Build history of the part. All positions in model axes, mm. A direction names the side the tool comes from. Give positions to 0.01 mm unless a question says otherwise; leave off trailing zeros. Write each loop counter-clockwise with the first axis right and the second up, starting at its lowest first coordinate (ties: lowest second). Pieces come first, ordered by that corner, then holes. Notation, with made-up numbers: M 25.5,87.25 L 35.5,87.25 A16 ccw 35.5,113.25 Z; hole C 32.25,31.5 d5. An arc over 180 degrees is marked long. Return JSON: item names as keys, results as strings. Group by question number.
Q1. Band-saw the part on B-B, the plane x = 36.5. Give the cut face in (y, z), then the cut area to 3 significant figures.
Q2. Tool access for faces 1 (the flat face through (103, 47, -1)), 2 (the flat face through (47, 8, -63)), 3 (the flat face through (105.81, 27.69, -66.84)): list every direction of +Z, -Z, +X, -X, +Y, -Y with a clear straight run to the whole face (end or side of a thin tool).
Q3. Band-saw the part on C-C, the plane z = -31.5. Give the cut face in (x, y), then the cut area to 3 significant figures.
Q4. Band-saw the part on A-A, the plane z = -13. Give the cut face in (x, y), then the cut area to 3 significant figures.
Q5. Band-saw the part on D-D, the plane z = 3.5. Give the cut face in (x, y), then the cut area to 3 significant figures.
Q6. Wall check: probe 1 along Z at (x, y) = (2, 9); probe 2 along X at (y, z) = (8.5, -52.5); probe 3 along Z at (x, y) = (85, 33). Give the ranges that are in metal, low to high.
Q7. Flat gauge pins, fed straight in: pin 1 Ø4 at (x, z) = (95, -59.01) entering from +Y; pin 2 Ø2 at (y, z) = (1, -43) entering from +X; pin 3 Ø6 at (x, z) = (44, -48) entering from -Y. Where does each tip first touch, or does it go through?
Q8. Pull direction X, two halves, no side cores. Call faces 4 (the flat face through (-11.06, 27.692, 1.698)), 5 (the flat face through (0, 3, -6)), 6 (the flat face through (37, 50, 2)), 7 (the flat face through (104.581, 3.042, -0.864)): +X half, -X half, draft (parallel to the pull), parting line (faces both ways), or undercut.
Autodesk Inventor part; units mm, degrees
ref_plane "YZ Plane" through (0, 0, 0) normal (1, 0, 0) x (0, 1, 0)
ref_plane "XZ Plane" through (0, 0, 0) normal (0, 1, 0) x (-1, 0, 0)
ref_plane "XY Plane" through (0, 0, 0) normal (0, 0, 1) x (1, 0, 0)
sketch "Sketch1" plane through (0, 0, 0) normal (0, 1, 0) x (-1, 0, 0)
  line L0 (0, 0) -> (-95, 0)
  line L1 (-95, 0) -> (-95, -65)
  line L2 (-95, -65) -> (0, -65)
  line L3 (0, -65) -> (0, 0)
  line L4 (0, -65) -> (12.9904, -57.5)
  line L5 (12.9904, -57.5) -> (12.9904, -7.5)
  line L6 (12.9904, -7.5) -> (0, 0)
  line L7 (-95, -65) -> (-107.9904, -57.5)
  line L8 (-107.9904, -57.5) -> (-107.9904, -7.5)
  line L9 (-107.9904, -7.5) -> (-95, 0)
  dimension "d0" = 95
  dimension "d1" = 65
  dimension "d2" = 15
  dimension "d3" = 15
  dimension "d4" = 120
  dimension "d5" = 15
  dimension "d6" = 15
  dimension "d7" = 120
extrude "Extrusion1" add sketch "Sketch1" along normal blind 5
sketch "Sketch2" plane through (0, 5, 0) normal (0, 1, 0) x (1, 0, 0)
  line L0 (1.0001, 63.5) -> (94.0001, 63.5)
  line L1 (94.0001, 63.5) -> (94.0001, 1.5)
  line L2 (94.0001, 1.5) -> (1.0001, 1.5)
  line L3 (1.0001, 1.5) -> (1.0001, 63.5)
  line L4 (0, 0) -> (95, 0)
  line L5 (-12.9904, 57.5) -> (-12.9904, 7.5)
  dimension "d10" = 93
  dimension "d11" = 62
  dimension "d12" = 1.5
  dimension "d13" = 13.9905
extrude "Extrusion2" add sketch "Sketch2" along normal blind 14
sketch "Sketch4" plane through (0, 5, 0) normal (0, 1, 0) x (1, 0, 0)
  line L0 (-12.9904, 57.5) -> (-12.9904, 7.5)
  line L1 (-12.9904, 57.5) -> (-12.9904, 7.5)
  line L2 (-12.9904, 7.5) -> (0, 0)
  line L3 (0, 0) -> (95, 0)
  line L4 (95, 0) -> (107.9904, 7.5)
  line L5 (95, 0) -> (107.9904, 7.5)
  line L6 (107.9904, 7.5) -> (107.9904, 57.5)
  line L7 (107.9904, 57.5) -> (95, 65)
  line L8 (107.9904, 57.5) -> (95, 65)
  line L9 (95, 65) -> (0, 65)
  line L10 (95, 65) -> (0, 65)
  line L11 (0, 65) -> (-12.9904, 57.5)
  line L12 (-19.9904, 61.5415) -> (-19.9904, 3.4585)
  line L13 (114.9904, 61.5415) -> (114.9904, 3.4585)
  line L14 (-1.8756, 72) -> (96.8756, 72)
  line L15 (-19.9904, 61.5415) -> (-1.8756, 72)
  line L16 (96.8756, 72) -> (114.9904, 61.5415)
  line L17 (114.9904, 3.4585) -> (96.8756, -7)
  line L18 (-19.9904, 3.4585) -> (-1.8756, -7)
  line L19 (-1.8756, -7) -> (96.8756, -7)
  line L20 (95, 0) -> (107.9904, 7.5)
  line L21 (107.9904, 7.5) -> (107.9904, 57.5)
  line L22 (0, 0) -> (95, 0)
  dimension "d22" = 7
  dimension "d23" = 7
  dimension "d24" = 7
  dimension "d25" = 7
  dimension "d26" = 7
  dimension "d27" = 7
  dimension "d28" = 7
  dimension "d29" = 7
extrude "Extrusion4" add sketch "Sketch4" along normal blind 45 and the other way blind 5
sketch "Sketch5" plane through (0, 0, 0) normal (0, -1, 0) x (1, 0, 0)
  line L0 (2.4999, -63) -> (92.4999, -63)
  line L1 (92.4999, -63) -> (92.4999, -2)
  line L2 (92.4999, -2) -> (2.4999, -2)
  line L3 (2.4999, -2) -> (2.4999, -63)
  line L4 (0, 0) -> (95, 0)
  line L5 (-12.9904, -57.5) -> (-12.9904, -7.5)
  line L6 (96.8756, 7) -> (-1.8756, 7)
  line L7 (114.9904, -61.5415) -> (114.9904, -3.4585)
  dimension "d34" = 61
  dimension "d35" = 90
  dimension "d43" = 9
  dimension "d44" = 22.4905
extrude "Extrusion5" cut sketch "Sketch5" against normal blind 16
chamfer "Chamfer1" distance 6 angle 45 8 edges at (47.5, 0, -72) (105.933, 0, -66.7707) (114.9904, 0, -32.5) (105.933, 0, 1.7707) (47.5, 0, 7) (-10.933, 0, 1.7707) (-19.9904, 0, -32.5) (-10.933, 0, -66.7707)
sketch "Sketch6" plane through (0, 0, 0) normal (0, -1, 0) x (1, 0, 0)
  line L0 (2.4999, -2) -> (-2.5001, -2)
  line L1 (-2.5001, -2) -> (-2.5001, -63.0139)
  line L2 (-2.5001, -63.0139) -> (2.4999, -63.0139)
  line L3 (2.4999, -63.0139) -> (2.4999, -2)
  line L4 (2.4999, -2) -> (92.4999, -2)
  line L5 (92.4999, -2) -> (97.4999, -2)
  line L6 (97.4999, -2) -> (97.4999, -63.0139)
  line L7 (97.4999, -63.0139) -> (92.4999, -63.0139)
  line L8 (92.4999, -63.0139) -> (92.4999, -2)
  point P0 (0, 0)
  dimension "d45" = 5
  dimension "d46" = 5
extrude "Extrusion6" cut sketch "Sketch6" against normal blind 2
sketch "Sketch7" plane through (0, 2, 0) normal (0, -1, 0) x (1, 0, 0)
  circle A0 centre (-0.0001, -6) radius 1.6
  circle A1 centre (94.9999, -6) radius 1.6
  circle A2 centre (-0.0001, -59.0139) radius 1.6
  circle A3 centre (94.9999, -59.0139) radius 1.6
  line L0 (94.0001, -63.5) -> (94.0001, -1.5)
  line L1 (2.4999, -2) -> (2.4999, -63)
  line L2 (97.4999, -2) -> (97.4999, -63.0139)
  line L3 (-2.5001, -2) -> (97.4999, -2)
  line L4 (-2.5001, -63.0139) -> (-2.5001, -2)
  line L5 (2.4999, -63.0139) -> (-2.5001, -63.0139)
  line L6 (92.4999, -63) -> (92.4999, -2)
  line L7 (97.4999, -63.0139) -> (92.4999, -63.0139)
  point P0 (0, 0)
  dimension "d49" = 3.2
  dimension "d50" = 2.5
  dimension "d51" = 2.5
  dimension "d52" = 4
  dimension "d53" = 0
  dimension "d54" = 2.5
  dimension "d55" = 4
  dimension "d56" = 2.5
  dimension "d57" = 4
extrude "Extrusion7" cut sketch "Sketch7" against normal blind 1 contours A0 | A1 L0 | L0 A1 | L0 A3 | A3 L0 | A2
sketch "Sketch8" plane through (0, 19, 0) normal (0, 1, 0) x (1, 0, 0)
  line L0 (5.0001, 60.5) -> (90.0001, 60.5)
  line L1 (90.0001, 60.5) -> (90.0001, 4.5)
  line L2 (90.0001, 4.5) -> (5.0001, 4.5)
  line L3 (5.0001, 4.5) -> (5.0001, 60.5)
  line L4 (96.8756, 72) -> (-1.8756, 72)
  line L5 (-19.9904, 61.5415) -> (-19.9904, 3.4585)
  circle A0 centre (28.5001, 57) radius 2.5
  circle A1 centre (28.5001, 8) radius 2.5
  circle A2 centre (86.5001, 57) radius 2.5
  circle A3 centre (86.5001, 8) radius 2.5
  point P0 (0, 0)
  dimension "d60" = 85
  dimension "d61" = 56
  dimension "d62" = 11.5
  dimension "d63" = 24.9905
  dimension "d65" = 3.5
  dimension "d66" = 5
  dimension "d68" = 3.5
  dimension "d69" = 3.5
  dimension "d70" = 3.5
  dimension "d71" = 58
  dimension "d72" = 58
  dimension "d75" = 3.5
  dimension "d76" = 3.5
extrude "Extrusion8" add sketch "Sketch8" along normal blind 5 contours A0 | A1 | A2 | A3
sketch "Sketch9" plane through (92.4999, 16, -63) normal (-1, 0, 0) x (0, 0, 1)
  circle A0 centre (49, -5) radius 3.5
  line L0 (61, 0) -> (0, 0)
  line L1 (61, -14) -> (61, 0)
  point P0 (63, -16)
  dimension "d77" = 7
  dimension "d78" = 5
  dimension "d79" = 12
extrude "Extrusion9" cut sketch "Sketch9" against normal blind 5
sketch "Sketch10" plane through (0, 50, 0) normal (0, 1, 0) x (1, 0, 0)
  line L0 (-12.9904, 7.5) -> (-12.9904, 57.5)
  line L1 (-12.9904, 7.5) -> (-16.4904, 1.4378)
  line L2 (-1.8756, -7) -> (-19.9904, 3.4585)
  line L3 (0, 0) -> (95, 0)
  line L4 (0, 0) -> (-3.486, -6.038)
  line L5 (-12.9904, 57.5) -> (0, 65)
  line L6 (-12.9904, 57.5) -> (-16.4904, 63.5622)
  line L7 (-1.8756, 72) -> (-19.9904, 61.5415)
  line L8 (0, 65) -> (-3.5, 71.0622)
  line L9 (0, 65) -> (95, 65)
  line L10 (95, 65) -> (98.5, 71.0622)
  line L11 (114.9904, 61.5415) -> (96.8756, 72)
  line L12 (107.9904, 57.5) -> (95, 65)
  line L13 (107.9904, 57.5) -> (111.4904, 63.5622)
  line L14 (95, 0) -> (107.9904, 7.5)
  line L15 (107.9904, 7.5) -> (111.4904, 1.4378)
  line L16 (95, 0) -> (98.5, -6.0622)
  line L17 (96.8756, -7) -> (114.9904, 3.4585)
  circle A0 centre (103.2452, 0.7189) radius 1.6
  circle A1 centre (103.2452, 64.2811) radius 1.6
  circle A2 centre (-8.2452, 64.2811) radius 1.6
  circle A3 centre (-8.2452, 0.7189) radius 1.6
  circle A4 centre (46.5, -3.5) radius 1.6
  circle A5 centre (46.5, 68.5) radius 1.6
  line L18 (0, 0) -> (-12.9904, 7.5)
  line L19 (-12.9904, 7.5) -> (0, 0)
  line L20 (0, 0) -> (0, -7)
  line L21 (-1.8756, -7) -> (96.8756, -7)
  line L22 (0, 65) -> (0, 72)
  dimension "d82" = 3.2
  dimension "d83" = 7.5
  dimension "d84" = 90
  dimension "d85" = 3.5
  dimension "d86" = 90
  dimension "d87" = 7.5
  dimension "d88" = 3.5
  dimension "d89" = 7.5
  dimension "d90" = 3.5
  dimension "d91" = 7.5
  dimension "d92" = 3.5
  dimension "d93" = 46.5
  dimension "d95" = 46.5
  dimension "d96" = 3.5
  dimension "d97" = 3.5
extrude "Extrusion10" cut sketch "Sketch10" against normal blind 3 contours A0 | A1 | A2 | A3 | A4 | A5
properties part number "Bottomv3"
From the geometry:
{
 "1": {"outline": "M 0,-66 L 6,-72 L 50,-72 L 50,-65 L 5,-65 L 5,-63.5 L 19,-63.5 L 19,-1.5 L 5,-1.5 L 5,0 L 50,0 L 50,7 L 6,7 L 0,1 L 0,-2 L 16,-2 L 16,-63 L 0,-63 Z", "area": "881 mm^2"},
 "2": {"face 1": "+Y", "face 2": "-Y", "face 3": "-Z, +X, +Y, -Y"},
 "3": {"outline": "M -19.99,6 L -13.99,0 L -2.5,0 L -2.5,2 L 2.5,2 L 2.5,16 L 92.5,16 L 92.5,2 L 97.5,2 L 97.5,0 L 108.99,0 L 114.99,6 L 114.99,50 L 107.99,50 L 107.99,5 L 94,5 L 94,19 L 1,19 L 1,5 L -12.99,5 L -12.99,50 L -19.99,50 Z", "area": "1,110 mm^2"},
 "4": {"outline": "M -19.99,6 L -13.99,0 L -2.5,0 L -2.5,2 L 2.5,2 L 2.5,16 L 92.5,16 L 92.5,14.35 L 94,14.35 L 94,19 L 1,19 L 1,5 L -12.99,5 L -12.99,50 L -19.99,50 Z; M 92.5,2 L 97.5,2 L 97.5,0 L 108.99,0 L 114.99,6 L 114.99,50 L 107.99,50 L 107.99,5 L 94,5 L 94,7.65 L 92.5,7.65 Z", "area": "1,100 mm^2"},
 "5": {"outline": "M -7.94,6 L -0.94,2.5 L 95.94,2.5 L 102.94,6 L 102.94,50 L 48.1,50 L 48.1,47 L 44.9,47 L 44.9,50 L -7.94,50 Z", "area": "5,230 mm^2"},
 "6": {"probe 1": "z = -72 to -65, -63.5 to -1.5, 0 to 7", "probe 2": "x = -19.99 to -12.99, 1 to 2.5, 92.5 to 94, 107.99 to 114.99", "probe 3": "z = -72 to -65, 0 to 7"},
 "7": {"pin 1": "stops at y = 19", "pin 2": "stops at x = 110.99", "pin 3": "stops at y = 16"},
 "8": {"face 4": "-X half", "face 5": "undercut", "face 6": "draft", "face 7": "+X half"}
}
